```python
from build123d import *

# Parameters (mm, degrees)
SKETCH1_R           = 2.399999999999999
SKETCH1_R_2         = 1.75
BOSS_EXTRUDE1_DEPTH = 5
FILLET1_R           = 2


with BuildPart() as part:
    # Sketch1 → Boss-Extrude1 (new body)
    with BuildSketch(Plane.XY):
        with BuildLine():
            Line((-5.500000000000002, 3.5), (5.499999999999998, 3.5))
            ThreePointArc((5.499999999999998, 3.5), (6.914213562373094, 2.914213562373095), (7.499999999999998, 1.4999999999999998))
            Line((7.499999999999998, 1.4999999999999998), (7.499999999999998, -1.5000000000000002))
            ThreePointArc((7.499999999999998, -1.5000000000000002), (6.914213562373094, -2.914213562373096), (5.499999999999998, -3.500000000000001))
            Line((5.499999999999998, -3.500000000000001), (-5.500000000000002, -3.500000000000001))
            ThreePointArc((-5.500000000000002, -3.500000000000001), (-6.914213562373097, -2.914213562373096), (-7.500000000000002, -1.5000000000000007))
            Line((-7.500000000000002, -1.5000000000000007), (-7.500000000000002, 1.4999999999999993))
            ThreePointArc((-7.500000000000002, 1.4999999999999993), (-6.914213562373097, 2.914213562373095), (-5.500000000000002, 3.5))
        make_face()
        with Locations((-3.5000000000000013, 0)):
            Circle(SKETCH1_R, mode=Mode.SUBTRACT)
        with Locations((3.5000000000000013, 1.29e-15)):
            Circle(SKETCH1_R_2, mode=Mode.SUBTRACT)
    extrude(amount=BOSS_EXTRUDE1_DEPTH)

    # Fillet1
    # the kernel refuses this fillet: 2 mm, written as the material it takes off along each edge
    with BuildSketch(Plane(origin=(-5.500000000000001, 1.4999999999999987, 5), x_dir=(-1, 3.3e-16, 0), z_dir=(-3.3e-16, -1, 0))) as fillet1_piece_1:
        with BuildLine():
            CenterArc((2.000000000000001 - FILLET1_R, FILLET1_R), FILLET1_R, 270, 90)
            Line((2.000000000000001 - FILLET1_R, 0), (2.000000000000001, 0))
            Line((2.000000000000001, 0), (2.000000000000001, FILLET1_R))
        make_face()
    revolve(axis=Axis((-5.500000000000001, 1.4999999999999987, 5), (0, 0, -1)), revolution_arc=89.99999999999996, mode=Mode.SUBTRACT)
    with BuildSketch(Plane(origin=(-7.500000000000002, -1.5000000000000007, 5), x_dir=(0, 0, -1), z_dir=(0, 1, 0)), Plane(origin=(7.499999999999998, 1.4999999999999998, 5), x_dir=(0, 0, -1), z_dir=(0, -1, 0))) as fillet1_piece_2:
        with BuildLine():
            CenterArc((FILLET1_R, -FILLET1_R), FILLET1_R, 90, 90)
            Line((0, -FILLET1_R), (0, 0))
            Line((0, 0), (FILLET1_R, 0))
        make_face()
    extrude(amount=3, mode=Mode.SUBTRACT)
    with BuildSketch(Plane(origin=(-5.500000000000002, -1.5000000000000002, 5), x_dir=(0, -1, 0), z_dir=(1, 0, 0))) as fillet1_piece_3:
        with BuildLine():
            CenterArc((2.000000000000001 - FILLET1_R, FILLET1_R), FILLET1_R, 270, 90)
            Line((2.000000000000001 - FILLET1_R, 0), (2.000000000000001, 0))
            Line((2.000000000000001, 0), (2.000000000000001, FILLET1_R))
        make_face()
    revolve(axis=Axis((-5.500000000000002, -1.5000000000000002, 5), (0, 0, -1)), revolution_arc=89.99999999999999, mode=Mode.SUBTRACT)
    with BuildSketch(Plane(origin=(5.499999999999998, -3.500000000000001, 5), x_dir=(0, 0, -1), z_dir=(-1, 0, 0)), Plane(origin=(-5.500000000000002, 3.5, 5), x_dir=(0, 0, -1), z_dir=(1, 0, 0))) as fillet1_piece_4:
        with BuildLine():
            CenterArc((FILLET1_R, -FILLET1_R), FILLET1_R, 90, 90)
            Line((0, -FILLET1_R), (0, 0))
            Line((0, 0), (FILLET1_R, 0))
        make_face()
    extrude(amount=11, mode=Mode.SUBTRACT)
    with BuildSketch(Plane(origin=(5.499999999999999, -1.5000000000000018, 5), x_dir=(1, 7.8e-16, 0), z_dir=(-7.8e-16, 1, 0))) as fillet1_piece_5:
        with BuildLine():
            CenterArc((1.9999999999999991 - FILLET1_R, FILLET1_R), FILLET1_R, 270, 90)
            Line((1.9999999999999991 - FILLET1_R, 0), (1.9999999999999991, 0))
            Line((1.9999999999999991, 0), (1.9999999999999991, FILLET1_R))
        make_face()
    revolve(axis=Axis((5.499999999999999, -1.5000000000000018, 5), (0, 0, -1)), revolution_arc=90.00000000000007, mode=Mode.SUBTRACT)
    with BuildSketch(Plane(origin=(5.499999999999999, 1.5000000000000013, 5), x_dir=(-4.4e-16, 1, 0), z_dir=(-1, -4.4e-16, 0))) as fillet1_piece_6:
        with BuildLine():
            CenterArc((1.9999999999999987 - FILLET1_R, FILLET1_R), FILLET1_R, 270, 90)
            Line((1.9999999999999987 - FILLET1_R, 0), (1.9999999999999987, 0))
            Line((1.9999999999999987, 0), (1.9999999999999987, FILLET1_R))
        make_face()
    revolve(axis=Axis((5.499999999999999, 1.5000000000000013, 5), (0, 0, -1)), revolution_arc=90.00000000000007, mode=Mode.SUBTRACT)


solid = part.part
```
Input: part model. Units: mm. Frame: model coordinates. Round coordinates to 2 decimals unless told otherwise and drop trailing zeros. Loops run counter-clockwise (first coordinate to the right, second up) from the corner with the lowest first, then second, coordinate; pieces in that order, holes last.
1) Section query B-B on y = 0. Return the cut outline in (x, z).
Ans:
outline: (-7.5, 0) - (-5.9, 0) - (-5.9, 4.96) arc R2 ccw to (-7.5, 3) - close; (-1.1, 0) - (1.75, 0) - (1.75, 5) - (-1.1, 5) - close; (5.25, 0) - (7.5, 0) - (7.5, 3) arc R2 ccw to (5.5, 5) - (5.25, 5) - close
2) Section query A-A on x = 3.25. Return the cut outline in (y, z), plus the area to 3 significant figures.
Ans:
outline: (-3.5, 0) - (-1.73, 0) - (-1.73, 4.99) arc R2 ccw to (-3.5, 3) - close; (1.73, 0) - (3.5, 0) - (3.5, 3) arc R2 ccw to (1.73, 4.99) - close
area: 16.0 mm2
3) Section query D-D on y = 2. Return the cut outline in (x, z).
Ans:
outline: (-7.44, 0) - (-4.83, 0) - (-4.83, 4.94) - (-5.5, 4.94) arc R1.94 ccw to (-7.44, 3) - close; (-2.17, 0) - (7.44, 0) - (7.44, 3) arc R1.94 ccw to (5.5, 4.94) - (-2.17, 4.94) - close
4) Section query C-C on z = 2.3. Return the cut outline in (x, y), plus the area to 3 significant figures.
Ans:
outline: (-7.5, -1.5) arc R2 ccw to (-5.5, -3.5) - (5.5, -3.5) arc R2 ccw to (7.5, -1.5) - (7.5, 1.5) arc R2 ccw to (5.5, 3.5) - (-5.5, 3.5) arc R2 ccw to (-7.5, 1.5) - close; hole circle Ø4.8 at (-3.5, 0); hole circle Ø3.5 at (3.5, 0)
area: 73.8 mm2
5) Pull-direction query (Y, two-part tool) for faces 1 (the flat face through (1, 0, 5)), 2 (the cylindrical face through (-1.21, 0.72, 2.46)), 3 (the cylindrical face through (-6.9, -2.93, 1.48)); classes: released by +Y, released by -Y, zero draft, split by the parting line, or undercut.
Ans:
face 1: zero draft
face 2: undercut
face 3: released by -Y
6) Material intervals for line 1 (Y direction, x = 3.5, z = 3.1); line 2 (X direction, y = 1, z = 2.6); line 3 (X direction, y = 0.5, z = 3.75), sorted ascending.
Ans:
line 1: y = -3.5 to -1.75, 1.75 to 3.5
line 2: x = -7.5 to -5.68, -1.32 to 2.06, 4.94 to 7.5
line 3: x = -7.35 to -5.85, -1.15 to 1.82, 5.18 to 7.35
